Model file for the job. Use its own axes, mm. A direction names the side the tool comes from. Coordinates: 2 decimals unless noted, no trailing zeros. Write each loop counter-clockwise with the first axis right and the second up, starting at its lowest first coordinate (ties: lowest second). Pieces come first, ordered by that corner, then holes. Notation, with made-up numbers: (18.5, -29.75) - (76.5, -29.75) arc R12 cw to (76.5, -13.75) - close; hole circle Ø7 at (35.25, -24). An arc over 180 degrees is marked (long way). Put each result on its own line as item: value. Start each with the question number.
1. Drop flat-ended pins along their axis: P1, Ø6, axis at x = 5.5, z = 5, coming from the +Y side; P2, Ø5, axis at x = -9.5, z = 4.5, coming from the +Y side (3 decimals); P3, Ø1, axis at x = -12.5, z = 4.5, coming from the +Y side. Give the stop position or say it passes through.
2. Saw through at C-C, the plane z = 3.25. Write the cut outline in (x, y), plus the area to 3 significant figures.
3. Which spindle directions (+Z, -Z, +X, -X, +Y, -Y) get a long thin tool onto all of the face, cutting with end or side? Do faces 1 (the face through (-17, 11, 1)), 2 (the face through (0, -9, 11)). Say none if no direction does.
4. Saw through at D-D, the plane y = -18. Write the cut outline in (x, z).
5. Drill centre lines: L1, parallel to Y at x = 0, z = 7.25; L2, parallel to Z at x = 23, y = 8; L3, parallel to Y at x = -6, z = 4. Where is each one in solid material? Low to high. Write a range as from..to.
6. Saw through at A-A, the plane y = 0. Write the cut outline in (x, z).
7. Pull direction X, two halves, no side cores. Call faces 3 (the face through (-7.493, 0.33, 6.07)), 4 (the face through (0, 0, 0)), 5 (the face through (0, 0, 1)), 6 (the face through (-4.336, -19.524, 5.93)): released by +X, released by -X, zero draft, split by the parting line, or undercut.
```python
from build123d import *

# Parameters (mm, degrees)
F0_W     = 50
F0_H     = 50
F1_DEPTH = 1
F2_R     = 20
F3_DEPTH = 10
F4_R     = 7.5
F5_DEPTH = 10


with BuildPart() as f1:
    # F0 (on Top) → F1 (new body)
    with BuildSketch(Plane.XY):
        Rectangle(F0_W, F0_H)
    extrude(amount=F1_DEPTH)

    # F2 (on face) → F3 (join)
    with BuildSketch(Plane.XY.offset(1)):
        Circle(F2_R)
    extrude(amount=F3_DEPTH)

    # F4 (on face) → F5 (cut)
    with BuildSketch(Plane.XY.offset(11)):
        Circle(F4_R)
    extrude(amount=-F5_DEPTH, mode=Mode.SUBTRACT)


solid = f1.part
```
Final values:
1. P1: stops at y = 19.84
1. P2: stops at y = 18.735
1. P3: stops at y = 16
2. outline: circle Ø40 at (0, 0); hole circle Ø15 at (0, 0)
2. area: 1,080 mm²
3. face 1: +Z
3. face 2: +Z, +X, -X, +Y, -Y
4. outline: (-25, 0) - (25, 0) - (25, 1) - (8.72, 1) - (8.72, 11) - (-8.72, 11) - (-8.72, 1) - (-25, 1) - close
5. L1: y = -20..-7.5, 7.5..20
5. L2: z = 0..1
5. L3: y = -19.08..-4.5, 4.5..19.08
6. outline: (-25, 0) - (25, 0) - (25, 1) - (20, 1) - (20, 11) - (7.5, 11) - (7.5, 1) - (-7.5, 1) - (-7.5, 11) - (-20, 11) - (-20, 1) - (-25, 1) - close
7. face 3: undercut
7. face 4: zero draft
7. face 5: undercut
7. face 6: split by the parting line
